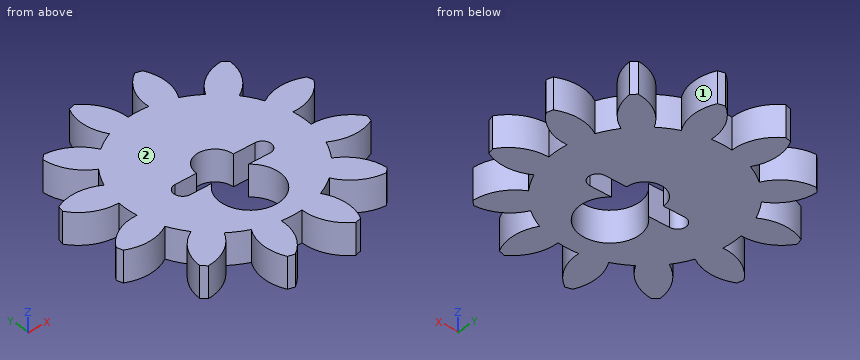
from build123d import *

# Parameters (mm, degrees)
BOSS_EXTRUDE1_DEPTH = 2.54


with BuildPart() as part:
    # Sketch1 → Boss-Extrude1 (new body)
    with BuildSketch(Plane.XY):
        with BuildLine():
            ThreePointArc((-7.372965122, 7.75726334), (-7.56755407, 7.56755407), (-7.75726334, 7.372965122))
            ThreePointArc((-7.75726334, 7.372965122), (-7.183443639, 5.605840676), (-5.817551904, 4.346341719))
            ThreePointArc((-5.817551904, 4.346341719), (-6.288954394, 3.630929512), (-6.672818294, 2.864976877))
            ThreePointArc((-6.672818294, 2.864976877), (-8.446522255, 3.41812434), (-10.263806767, 3.031504555))
            ThreePointArc((-10.263806767, 3.031504555), (-10.337471104, 2.769917034), (-10.404469677, 2.506543427))
            ThreePointArc((-10.404469677, 2.506543427), (-9.023965016, 1.263078615), (-7.211318596, 0.85526639))
            ThreePointArc((-7.211318596, 0.85526639), (-7.261859025, 0), (-7.211318596, -0.85526639))
            ThreePointArc((-7.211318596, -0.85526639), (-9.023965016, -1.263078615), (-10.404469677, -2.506543427))
            ThreePointArc((-10.404469677, -2.506543427), (-10.337471104, -2.769917034), (-10.263806767, -3.031504555))
            ThreePointArc((-10.263806767, -3.031504555), (-8.446522255, -3.41812434), (-6.672818294, -2.864976877))
            ThreePointArc((-6.672818294, -2.864976877), (-6.288954394, -3.630929512), (-5.817551904, -4.346341719))
            ThreePointArc((-5.817551904, -4.346341719), (-7.183443639, -5.605840676), (-7.75726334, -7.372965122))
            ThreePointArc((-7.75726334, -7.372965122), (-7.56755407, -7.56755407), (-7.372965122, -7.75726334))
            ThreePointArc((-7.372965122, -7.75726334), (-5.605840676, -7.183443639), (-4.346341719, -5.817551904))
            ThreePointArc((-4.346341719, -5.817551904), (-3.630929512, -6.288954394), (-2.864976877, -6.672818294))
            ThreePointArc((-2.864976877, -6.672818294), (-3.41812434, -8.446522255), (-3.031504555, -10.263806767))
            ThreePointArc((-3.031504555, -10.263806767), (-2.769917034, -10.337471104), (-2.506543427, -10.404469677))
            ThreePointArc((-2.506543427, -10.404469677), (-1.263078615, -9.023965016), (-0.85526639, -7.211318596))
            ThreePointArc((-0.85526639, -7.211318596), (0, -7.261859025), (0.85526639, -7.211318596))
            ThreePointArc((0.85526639, -7.211318596), (1.263078615, -9.023965016), (2.506543427, -10.404469677))
            ThreePointArc((2.506543427, -10.404469677), (2.769917034, -10.337471104), (3.031504555, -10.263806767))
            ThreePointArc((3.031504555, -10.263806767), (3.41812434, -8.446522255), (2.864976877, -6.672818294))
            ThreePointArc((2.864976877, -6.672818294), (3.630929512, -6.288954394), (4.346341719, -5.817551904))
            ThreePointArc((4.346341719, -5.817551904), (5.605840676, -7.183443639), (7.372965122, -7.75726334))
            ThreePointArc((7.372965122, -7.75726334), (7.56755407, -7.56755407), (7.75726334, -7.372965122))
            ThreePointArc((7.75726334, -7.372965122), (7.183443639, -5.605840676), (5.817551904, -4.346341719))
            ThreePointArc((5.817551904, -4.346341719), (6.288954394, -3.630929512), (6.672818294, -2.864976877))
            ThreePointArc((6.672818294, -2.864976877), (8.446522255, -3.41812434), (10.263806767, -3.031504555))
            ThreePointArc((10.263806767, -3.031504555), (10.337471104, -2.769917034), (10.404469677, -2.506543427))
            ThreePointArc((10.404469677, -2.506543427), (9.023965016, -1.263078615), (7.211318596, -0.85526639))
            ThreePointArc((7.211318596, -0.85526639), (7.261859025, 0), (7.211318596, 0.85526639))
            ThreePointArc((7.211318596, 0.85526639), (9.023965016, 1.263078615), (10.404469677, 2.506543427))
            ThreePointArc((10.404469677, 2.506543427), (10.337471104, 2.769917034), (10.263806767, 3.031504555))
            ThreePointArc((10.263806767, 3.031504555), (8.446522255, 3.41812434), (6.672818294, 2.864976877))
            ThreePointArc((6.672818294, 2.864976877), (6.288954394, 3.630929512), (5.817551904, 4.346341719))
            ThreePointArc((5.817551904, 4.346341719), (7.183443639, 5.605840676), (7.75726334, 7.372965122))
            ThreePointArc((7.75726334, 7.372965122), (7.56755407, 7.56755407), (7.372965122, 7.75726334))
            ThreePointArc((7.372965122, 7.75726334), (5.605840676, 7.183443639), (4.346341719, 5.817551904))
            ThreePointArc((4.346341719, 5.817551904), (3.630929512, 6.288954394), (2.864976877, 6.672818294))
            ThreePointArc((2.864976877, 6.672818294), (3.41812434, 8.446522255), (3.031504555, 10.263806767))
            ThreePointArc((3.031504555, 10.263806767), (2.769917034, 10.337471104), (2.506543427, 10.404469677))
            ThreePointArc((2.506543427, 10.404469677), (1.263078615, 9.023965016), (0.85526639, 7.211318596))
            ThreePointArc((0.85526639, 7.211318596), (0, 7.261859025), (-0.85526639, 7.211318596))
            ThreePointArc((-0.85526639, 7.211318596), (-1.263078615, 9.023965016), (-2.506543427, 10.404469677))
            ThreePointArc((-2.506543427, 10.404469677), (-2.769917034, 10.337471104), (-3.031504555, 10.263806767))
            ThreePointArc((-3.031504555, 10.263806767), (-3.41812434, 8.446522255), (-2.864976877, 6.672818294))
            ThreePointArc((-2.864976877, 6.672818294), (-3.630929512, 6.288954394), (-4.346341719, 5.817551904))
            ThreePointArc((-4.346341719, 5.817551904), (-5.605840676, 7.183443639), (-7.372965122, 7.75726334))
        make_face()
        with BuildLine():
            Line((-1.524, -1.424354318), (-3.302, -1.424354318))
            ThreePointArc((-3.302, -1.424354318), (-4.014177159, -0.712177159), (-3.302, 0))
            Line((-3.302, 0), (-1.524, 0))
            ThreePointArc((-1.524, 0), (0, 1.524), (1.524, 0))
            Line((1.524, 0), (3.302, 0))
            ThreePointArc((3.302, 0), (4.014177159, -0.712177159), (3.302, -1.424354318))
            Line((3.302, -1.424354318), (1.524, -1.424354318))
            ThreePointArc((1.524, -1.424354318), (0, -5.70818114), (-1.524, -1.424354318))
        make_face(mode=Mode.SUBTRACT)
    extrude(amount=BOSS_EXTRUDE1_DEPTH)


solid = part.part
Geometry: final body of the model. Coordinates: model frame, mm. Face numbers are marked on the shaded views. Give positions to 0.01 mm unless a question says otherwise; leave off trailing zeros. Write each loop counter-clockwise with the first axis right and the second up, starting at its lowest first coordinate (ties: lowest second). Pieces come first, ordered by that corner, then holes. Notation, with made-up numbers: (-21, 67) -> (-14, 67) arc R31 ccw to (-14, 99) -> close; hole circle Ø3 at (61, 8.25). An arc over 180 degrees is marked (long way). Answer in a Markdown table with one row per item.
(1) Pin query (flat end, axial travel): pin 1 (4 mm diameter, centred on x = 0, y = -3.3, fed in from +Z); pin 2 (1.5 mm diameter, centred on x = -7.5, z = 1, fed in from -Y); pin 3 (0.5 mm diameter, centred on x = -2, z = 1, fed in from +Y); pin 4 (0.5 mm diameter, centred on x = -3, z = 1, fed in from -Y). Return the tip coordinate at first contact, or that it passes through.
Answers below:
| item | result |
|---|---|
| pin 1 | through |
| pin 2 | y = -7.76 |
| pin 3 | y = 10.22 |
| pin 4 | y = -10.34 |
(2) Section query B-B on x = 5.25. Return loops of the section in (y, z), then the cut area to 3 significant figures.
Answers below:
| item | result |
|---|---|
| outline | (-6.92, 0) -> (6.92, 0) -> (6.92, 2.54) -> (-6.92, 2.54) -> close |
| area | 35.2 mm^2 |
(3) Ray query, line 1 along X through (y, z) = (3, 1); line 2 along Y through (x, z) = (6.5, 1.3); line 3 along X through (y, z) = (-6.25, 0.9). Return the intervals inside material, ascending. Write a range as [from, to].
Answers below:
| item | result |
|---|---|
| line 1 | [-10.27, -6.91], [-6.61, 6.61], [6.91, 10.27] |
| line 2 | [-7.6, -4.82], [-3.24, 3.24], [4.82, 7.6] |
| line 3 | [-7.51, -4.62], [-3.7, 3.7], [4.62, 7.51] |
(4) Draft query along Y for the marked faces 1 and 2. Return one class per face: +Y half, -Y half, draft (parallel to the pull), parting line (faces both ways), or undercut.
Answers below:
| item | result |
|---|---|
| face 1 | undercut |
| face 2 | draft |
(5) Section query A-A on x = 0. Return loops of the section in (y, z).
Answers below:
| item | result |
|---|---|
| outline | (-7.26, 0) -> (-5.71, 0) -> (-5.71, 2.54) -> (-7.26, 2.54) -> close; (1.52, 0) -> (7.26, 0) -> (7.26, 2.54) -> (1.52, 2.54) -> close |
